Input: part model. Units: mm. Frame: model coordinates. A direction names the side the tool comes from. Round coordinates to 2 decimals unless told otherwise and drop trailing zeros. Order: outer loops, then holes, each group sorted by start corner. A loop starts at its lowest first (then second) coordinate and runs counter-clockwise, first axis right, second up.
Item 1: Cut plane B-B on y = 16.75. Output: boundary loops of the cut face in (x, z).
Item 2: First-contact query: pin 1 (10 mm diameter, centred on x = -30.5, y = 5.5, fed in from +Z); pin 2 (5 mm diameter, centred on y = 18, z = -5.5, fed in from -X); pin 3 (2 mm diameter, centred on y = 5, z = -7.5, fed in from -X); pin 4 (12 mm diameter, centred on x = -34.5, z = 7.5, fed in from -Y). Flat tips, straight axial feed; report the tip coordinate or a pass-through.
Item 3: Reachability of faces 4 (the cylindrical face through (-9.538, 12.58, 42.954)), 5 (the cylindrical face through (-10.04, 3.8, 45.2)) from +Z, -Z, +X, -X, +Y, -Y: full face, straight path, thin tool, end or side. Return the list, or none.
Item 4: Mould query, pull axis Y, two halves, no side actions, for faces 1 (the conical face through (20.44, 21.23, 39.3)), 2 (the flat face through (46.4, 1.6, -15.3)), 3 (the flat face through (33.3, 11.7, 30)). Classes: released by +Y, released by -Y, zero draft, split by the parting line, or undercut.
Item 5: Cut plane C-C on x = 0. Give the number of separate pieces and of enclosed holes in the cut face, then the cut area to 4 significant figures.
Item 6: Line query: L1, parallel to Z at x = 0, y = 12.45; L2, parallel to X at y = 5.75, z = 0; L3, parallel to Z at x = 0, y = 3.25. Output: solid intervals per line, ascending.
```python
from build123d import *

# Parameters (mm, degrees)
CUT_EXTRUDE1_REACH      = 79.324
CUT_EXTRUDE1_END_RADIUS = 47.3
SKETCH4_W               = 21
SKETCH4_H               = 6
FILLET1_R               = 2
FILLET2_R               = 0.5


with BuildPart() as part:
    # Sketch2 → Revolve1 (revolve)
    with BuildSketch(Plane.XY):
        Polygon((46.3, 0), (46.3, 21.6), (47.3, 21.6), (47.3, 1.6), (52.5, 1.6), (52.5, 0), align=None)
    revolve(axis=Axis((0, -1000, 0), (0, 1, 0)))

    # Cut-Extrude1: up to this cylinder (the profile starts inside it)
    cut_extrude1_end = Plane(origin=(0, 4.6, 0), z_dir=(0, -1, 0)) * Cylinder(CUT_EXTRUDE1_END_RADIUS, 254.248, mode=Mode.PRIVATE)
    # Sketch4 → Cut-Extrude1 (cut, up to the surface)
    with BuildSketch(Plane.XY, mode=Mode.PRIVATE) as cut_extrude1_sk1:
        with Locations((0, 4.6)):
            Rectangle(SKETCH4_W, SKETCH4_H)
    cut_extrude1_tool1 = extrude(cut_extrude1_sk1.sketch, amount=-CUT_EXTRUDE1_REACH, mode=Mode.PRIVATE) & cut_extrude1_end
    add(cut_extrude1_tool1.solids().sort_by_distance((0, 4.6, 0))[0], mode=Mode.SUBTRACT)

    # Fillet1
    fillet1_edges = [part.edges().sort_by_distance(p)[0] for p in [
        (10.5, 1.6, -45.606762076),
        (-10.5, 7.6, -45.606762076),
        (10.5, 7.6, -45.606762076),
        (-10.5, 1.6, -45.606762076),
    ]]
    fillet(fillet1_edges, radius=FILLET1_R)

    # Sketch6 → Revolve2 (revolve)
    with BuildSketch(Plane.XY, mode=Mode.PRIVATE) as revolve2_sk:
        Polygon((-46.3, 7.5), (-44.243032454, 21.6), (-46.3, 21.6), align=None)
        Polygon((-45.431988872, 13.45), (-45.687286263, 11.7), (-44, 11.7), (-44, 13.45), align=None)
    revolve(revolve2_sk.sketch.rotate(Axis((0, -1000, 0), (0, 1, 0)), 180), axis=Axis((0, -1000, 0), (0, 1, 0)))

    # Fillet2
    fillet2_edges = [part.edges().sort_by_distance(p)[0] for p in [
        (-45.687286263, 11.7, 0),
        (-44, 11.7, 0),
        (-44, 13.45, 0),
        (-45.431988872, 13.45, 0),
    ]]
    fillet(fillet2_edges, radius=FILLET2_R)

    # Sketch7 → Cut-Revolve1 (revolve, cut)
    with BuildSketch(Plane.XY):
        Polygon((-47.3, 1.6), (-47.3, 0.35), (-48.55, 1.6), align=None)
    revolve(axis=Axis((0, 0, 0), (0, 1, 0)), mode=Mode.SUBTRACT)


solid = part.part
```
From the geometry:
1. outline: circle Ø94.6 at (0, 0); hole circle Ø89.9 at (0, 0)
2. pin 1: stops at z = 44.8
2. pin 2: stops at x = -47.2
2. pin 3: stops at x = -46.85
2. pin 4: passes through
3. face 4: +Y, -Y
3. face 5: -Y
4. face 1: undercut
4. face 2: released by +Y
4. face 3: released by -Y
5. separate pieces: 3
5. enclosed holes: 0
5. area: 86.75 mm2
6. L1: z = -47.3 to -44, 44 to 47.3
6. L2: x = -47.3 to -46.3, 46.3 to 47.3
6. L3: z = 46.3 to 47.3
